Verification items for the finished model (mm, model axes). Coordinates: 2 decimals unless noted, no trailing zeros. Order: outer loops, then holes, each group sorted by start corner. A loop starts at its lowest first (then second) coordinate and runs counter-clockwise, first axis right, second up. Notation, with made-up numbers: (51.5, 76) -> (93.5, 76) arc R16 cw to (93.5, 81) -> close; hole circle Ø4 at (-9, 80). An arc over 180 degrees is marked (long way). Write each question's results on one line, items separated by ' | '. Start each with the question number.
(1) Cross-section at A-A on x = 204. Enter the section's corners in (y, z), and give its area (3 significant figures).
(2) Cross-section at C-C on z = 7.75. Enter the section's corners in (x, y).
(3) Cross-section at B-B on y = 38.5. Enter the section's corners in (x, z), and give its area (3 significant figures).
(4) Go/stop test with flat-tipped pins: pin 1 (1.5 mm diameter, centred on y = 29, z = 3, fed in from -X); pin 2 (4 mm diameter, centred on x = 88, z = 5, fed in from +Y); pin 3 (2.5 mm diameter, centred on y = 44.5, z = 6.5, fed in from +X). Record where each tip stops, or that it passes through.
(5) Thickness scan on probe 1 along X at (y, z) = (47, 8); probe 2 along Y at (x, z) = (199, 8.5); probe 3 along X at (y, z) = (19.5, 4.25). Record the ranges inside material, lowest first. Write a range as [from, to].
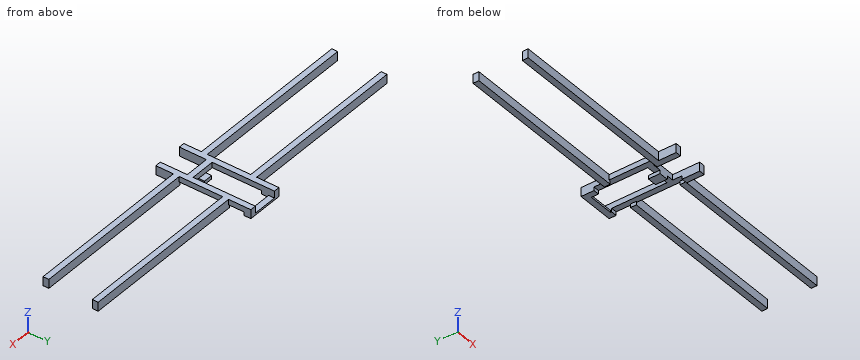
```python
from build123d import *

# Parameters (mm, degrees)
BOX012_W     = 8
BOX012_H     = 10
BOX012_DEPTH = 3
BOX013_W     = 146
BOX013_H     = 5
BOX013_DEPTH = 7.6
BOX014_W     = 146
BOX014_H     = 5
BOX014_DEPTH = 7.6
BOX015_W     = 146
BOX015_H     = 5
BOX015_DEPTH = 7.6
BOX016_W     = 146
BOX016_H     = 5
BOX016_DEPTH = 7.6
BOX009_W     = 5
BOX009_H     = 50
BOX009_DEPTH = 3
BOX010_W     = 5
BOX010_H     = 60
BOX010_DEPTH = 3
BOX011_W     = 22
BOX011_H     = 5
BOX011_DEPTH = 3
BOX006_W     = 5
BOX006_H     = 81
BOX006_DEPTH = 7.6
BOX007_W     = 22
BOX007_H     = 5
BOX007_DEPTH = 7.6
BOX008_W     = 22
BOX008_H     = 5
BOX008_DEPTH = 1.7
BOX005_W     = 5
BOX005_H     = 81
BOX005_DEPTH = 7.6


with BuildPart() as cube011:
    # Box012 → Box012 (new body)
    with BuildSketch(Plane(origin=(157, 23, 2), x_dir=(1, 0, 0), z_dir=(0, 0, 1))):
        with Locations((4, 5)):
            Rectangle(BOX012_W, BOX012_H)
    extrude(amount=BOX012_DEPTH)


with BuildPart() as cube012:
    # Box013 → Box013 (new body)
    with BuildSketch(Plane(origin=(0, 15, 2), x_dir=(1, 0, 0), z_dir=(0, 0, 1))):
        with Locations((73, 2.5)):
            Rectangle(BOX013_W, BOX013_H)
    extrude(amount=BOX013_DEPTH)


with BuildPart() as cube013:
    # Box014 → Box014 (new body)
    with BuildSketch(Plane(origin=(0, 57, 2), x_dir=(1, 0, 0), z_dir=(0, 0, 1))):
        with Locations((73, 2.5)):
            Rectangle(BOX014_W, BOX014_H)
    extrude(amount=BOX014_DEPTH)


with BuildPart() as cube014:
    # Box015 → Box015 (new body)
    with BuildSketch(Plane(origin=(175, 57, 2), x_dir=(1, 0, 0), z_dir=(0, 0, 1))):
        with Locations((73, 2.5)):
            Rectangle(BOX015_W, BOX015_H)
    extrude(amount=BOX015_DEPTH)


with BuildPart() as cube015:
    # Box016 → Box016 (new body)
    with BuildSketch(Plane(origin=(175, 15, 2), x_dir=(1, 0, 0), z_dir=(0, 0, 1))):
        with Locations((73, 2.5)):
            Rectangle(BOX016_W, BOX016_H)
    extrude(amount=BOX016_DEPTH)


with BuildPart() as cube008:
    # Box009 → Box009 (new body)
    with BuildSketch(Plane(origin=(134.4, 20, 2), x_dir=(1, 0, 0), z_dir=(0, 0, 1))):
        with Locations((2.5, 25)):
            Rectangle(BOX009_W, BOX009_H)
    extrude(amount=BOX009_DEPTH)


with BuildPart() as cube009:
    # Box010 → Box010 (new body)
    with BuildSketch(Plane(origin=(160.6, 15, 2), x_dir=(1, 0, 0), z_dir=(0, 0, 1))):
        with Locations((2.5, 30)):
            Rectangle(BOX010_W, BOX010_H)
    extrude(amount=BOX010_DEPTH)


with BuildPart() as cube010:
    # Box011 → Box011 (new body)
    with BuildSketch(Plane(origin=(139, 23, 2), x_dir=(1, 0, 0), z_dir=(0, 0, 1))):
        with Locations((11, 2.5)):
            Rectangle(BOX011_W, BOX011_H)
    extrude(amount=BOX011_DEPTH)


with BuildPart() as cube005:
    # Box006 → Box006 (new body)
    with BuildSketch(Plane(origin=(160.6, 0, 2), x_dir=(1, 0, 0), z_dir=(0, 0, 1))):
        with Locations((2.5, 40.5)):
            Rectangle(BOX006_W, BOX006_H)
    extrude(amount=BOX006_DEPTH)


with BuildPart() as cube006:
    # Box007 → Box007 (new body)
    with BuildSketch(Plane(origin=(139, 23, 2), x_dir=(1, 0, 0), z_dir=(0, 0, 1))):
        with Locations((11, 2.5)):
            Rectangle(BOX007_W, BOX007_H)
    extrude(amount=BOX007_DEPTH)


with BuildPart() as cube007:
    # Box008 → Box008 (new body)
    with BuildSketch(Plane(origin=(139, 76, 2), x_dir=(1, 0, 0), z_dir=(0, 0, 1))):
        with Locations((11, 2.5)):
            Rectangle(BOX008_W, BOX008_H)
    extrude(amount=BOX008_DEPTH)


with BuildPart() as holder:
    # Box005 → Box005 (new body)
    with BuildSketch(Plane(origin=(134.4, 0, 2), x_dir=(1, 0, 0), z_dir=(0, 0, 1))):
        with Locations((2.5, 40.5)):
            Rectangle(BOX005_W, BOX005_H)
    extrude(amount=BOX005_DEPTH)

    # Fusion003: union Cube005, Cube006, Cube007
    add(cube005.part)
    add(cube006.part)
    add(cube007.part)

    # Cut009: cut Cube010
    add(cube010.part, mode=Mode.SUBTRACT)

    # Cut010: cut Cube009
    add(cube009.part, mode=Mode.SUBTRACT)

    # Cut011: cut Cube008
    add(cube008.part, mode=Mode.SUBTRACT)


with BuildPart() as holder_1:
    # Cut011 placement: moved
    add(holder.part.moved(Location((10.5, 0, 0))))

    # Fusion004: union Cube011, Cube012, Cube013, Cube014, Cube015
    add(cube011.part)
    add(cube012.part)
    add(cube013.part)
    add(cube014.part)
    add(cube015.part)


solid = holder_1.part
```
Results are:
1) outline: (15, 2) -> (20, 2) -> (20, 9.6) -> (15, 9.6) -> close; (57, 2) -> (62, 2) -> (62, 9.6) -> (57, 9.6) -> close | area: 76.0 mm2
2) outline: (0, 15) -> (144.9, 15) -> (144.9, 0) -> (149.9, 0) -> (149.9, 23) -> (171.1, 23) -> (171.1, 0) -> (176.1, 0) -> (176.1, 15) -> (321, 15) -> (321, 20) -> (176.1, 20) -> (176.1, 57) -> (321, 57) -> (321, 62) -> (176.1, 62) -> (176.1, 81) -> (171.1, 81) -> (171.1, 28) -> (149.9, 28) -> (149.9, 81) -> (144.9, 81) -> (144.9, 62) -> (0, 62) -> (0, 57) -> (144.9, 57) -> (144.9, 20) -> (0, 20) -> close
3) outline: (144.9, 5) -> (149.9, 5) -> (149.9, 9.6) -> (144.9, 9.6) -> close; (171.1, 5) -> (176.1, 5) -> (176.1, 9.6) -> (171.1, 9.6) -> close | area: 46.0 mm2
4) pin 1: stops at x = 157 | pin 2: stops at y = 62 | pin 3: stops at x = 176.1
5) probe 1: x = [144.9, 149.9], [171.1, 176.1] | probe 2: y = [15, 20], [57, 62] | probe 3: x = [0, 149.9], [175, 321]
